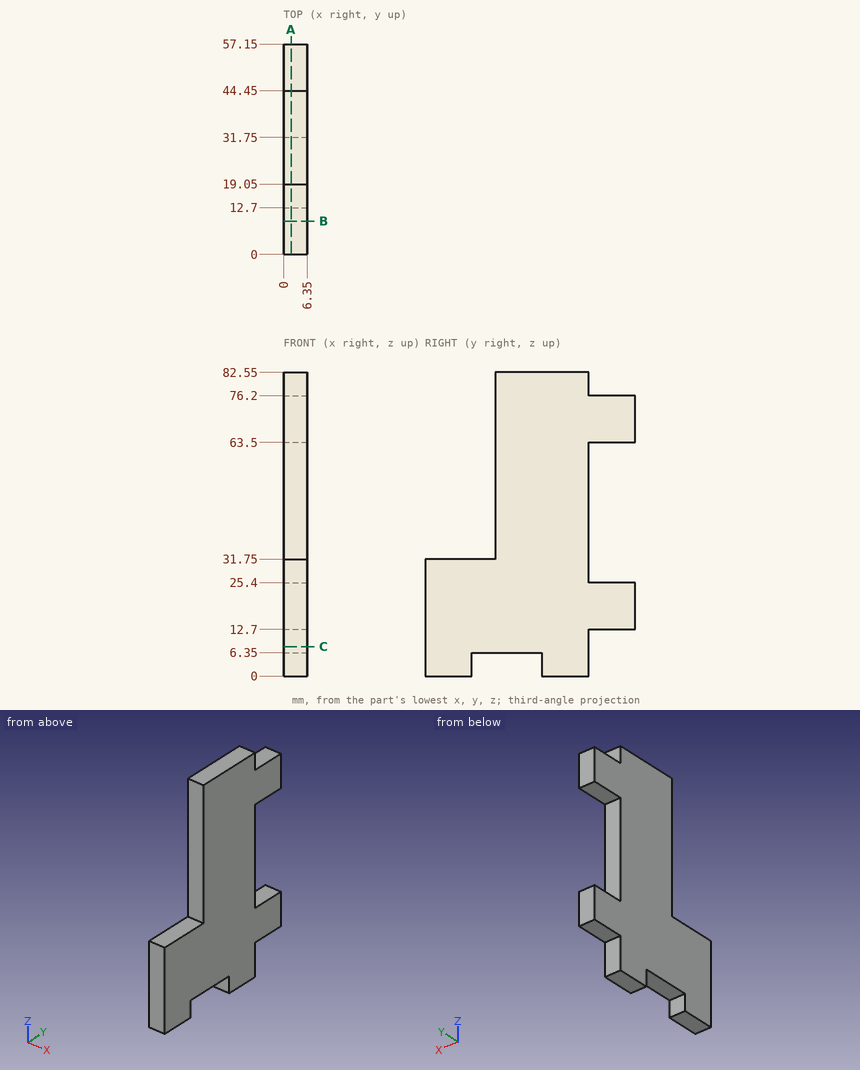
Check sheet for the drawn part. Datum: minimum x, y, z corner. Units: mm. Coordinates: 2 decimals unless noted, no trailing zeros. Order: outer loops, then holes, each group sorted by start corner. A loop starts at its lowest first (then second) coordinate and runs counter-clockwise, first axis right, second up. Notation, with made-up numbers: (-16.75, -5.5) - (36.25, -5.5) arc R28 ccw to (36.25, 21.5) - close; hole circle Ø4 at (39, 66). An arc over 180 degrees is marked (long way). Return JSON: item names as keys, results as strings.
(1) Section check B-B, the plane y = 9. Record the cut outline in (x, z).
Filled sheet:
{"outline": "(0, 0) - (6.35, 0) - (6.35, 31.75) - (0, 31.75) - close"}
(2) Section check A-A, the plane x = 2. Record the cut outline in (y, z), and give its area (3 significant figures).
Filled sheet:
{"outline": "(0, 0) - (12.7, 0) - (12.7, 6.35) - (31.75, 6.35) - (31.75, 0) - (44.45, 0) - (44.45, 12.7) - (57.15, 12.7) - (57.15, 25.4) - (44.45, 25.4) - (44.45, 63.5) - (57.15, 63.5) - (57.15, 76.2) - (44.45, 76.2) - (44.45, 82.55) - (19.05, 82.55) - (19.05, 31.75) - (0, 31.75) - close", "area": "2,900 mm^2"}
(3) Section check C-C, the plane z = 8. Record the cut outline in (x, y), and give its area (3 significant figures).
Filled sheet:
{"outline": "(0, 0) - (6.35, 0) - (6.35, 44.45) - (0, 44.45) - close", "area": "282 mm^2"}
(4) Thickness scan on line 1 along Z through (x, y) = (5, 45.5); line 2 along Y through (x, z) = (5.5, 37.5); line 3 along Z through (x, y) = (6, 12.5). Record the ranges inside material, lowest first.
Filled sheet:
{"line 1": "z = 12.7 to 25.4, 63.5 to 76.2", "line 2": "y = 19.05 to 44.45", "line 3": "z = 0 to 31.75"}
(5) Go/stop test with flat-tipped pins: pin 1 (3 mm diameter, centred on x = 4, y = 49.5, fed in from -Z); pin 2 (1.9 mm diameter, centred on x = 2.5, y = 48.5, fed in from +Z); pin 3 (1.9 mm diameter, centred on x = 2, z = 2, fed in from +Y). Record where each tip stops, or that it passes through.
Filled sheet:
{"pin 1": "stops at z = 12.7", "pin 2": "stops at z = 76.2", "pin 3": "stops at y = 44.45"}
